from build123d import *

# Parameters (mm, degrees)
BOSS_EXTRUDE1_DEPTH = 5
BOSS_EXTRUDE2_DEPTH = 40
CUT_EXTRUDE1_DEPTH  = 2
CUT_EXTRUDE2_DEPTH  = 370.382836634
FILLET1_R           = 18
FILLET2_R           = 7.5


with BuildPart() as part:
    # Sketch1 → Boss-Extrude1 (new body)
    with BuildSketch(Plane.XY):
        Polygon((67.7, -325.2), (75.2, -325.2), (75.2, -359.2), (-75.2, -359.2), (-75.2, -325.2), (-67.7, -325.2), (-67.7, -345.2), (67.7, -345.2), align=None)
    extrude(amount=-BOSS_EXTRUDE1_DEPTH)

    # Sketch2 → Boss-Extrude2 (add)
    with BuildSketch(Plane(origin=(0, 0, -5), x_dir=(-1, 0, 0), z_dir=(0, 0, -1))):
        Polygon((67.7, -325.2), (75.2, -325.2), (75.2, -359.2), (64.2, -359.2), (64.2, -345.2), (67.7, -345.2), align=None)
        Polygon((-75.2, -359.2), (-75.2, -325.2), (-67.7, -325.2), (-67.7, -345.2), (-64.2, -345.2), (-64.2, -359.2), align=None)
    extrude(amount=BOSS_EXTRUDE2_DEPTH)

    # Sketch3 → Cut-Extrude1 (cut)
    with BuildSketch(Plane(origin=(0, 0, -5), x_dir=(-1, 0, 0), z_dir=(0, 0, -1))):
        with BuildLine():
            Line((-29.2, -347.2), (30.8, -347.2))
            ThreePointArc((30.8, -347.2), (35.8, -352.2), (30.8, -357.2))
            Line((30.8, -357.2), (-29.2, -357.2))
            ThreePointArc((-29.2, -357.2), (-34.2, -352.2), (-29.2, -347.2))
        make_face()
    extrude(amount=-CUT_EXTRUDE1_DEPTH, mode=Mode.SUBTRACT)

    # Sketch4 → Cut-Extrude2 (cut, through all)
    with BuildSketch(Plane(origin=(0, 0, -3), x_dir=(-1, 0, 0), z_dir=(0, 0, -1))):
        with BuildLine():
            Line((-29.2, -349.2), (30.8, -349.2))
            ThreePointArc((30.8, -349.2), (33.8, -352.2), (30.8, -355.2))
            Line((30.8, -355.2), (-29.2, -355.2))
            ThreePointArc((-29.2, -355.2), (-32.2, -352.2), (-29.2, -349.2))
        make_face()
    extrude(amount=-CUT_EXTRUDE2_DEPTH, mode=Mode.SUBTRACT)

    # Fillet1
    fillet1_edges = [part.edges().sort_by_distance(p)[0] for p in [
        (-64.2, -352.2, -5),
        (64.2, -352.2, -5),
    ]]
    fillet(fillet1_edges, radius=FILLET1_R)

    # Fillet2
    fillet2_edges = [part.edges().sort_by_distance(p)[0] for p in [
        (75.2, -325.2, -22.5),
        (-75.2, -325.2, -22.5),
        (-75.2, -359.2, -22.5),
        (75.2, -359.2, -22.5),
    ]]
    fillet(fillet2_edges, radius=FILLET2_R - 0.0001)  # a hair under: the kernel refuses the full size


solid = part.part
Design review of the part built by this model. Coordinates are the model's own, in mm. A direction names the side the tool comes from. Coordinates: 2 decimals unless noted, no trailing zeros. Order: outer loops, then holes, each group sorted by start corner. A loop starts at its lowest first (then second) coordinate and runs counter-clockwise, first axis right, second up. Notation, with made-up numbers: (36.25, 64.25) - (47.25, 64.25) arc R21 cw to (47.25, 85.25) - close; hole circle Ø1 at (17, 40.5). An arc over 180 degrees is marked (long way). Put each result on its own line as item: value.
1) Tool access review of faces 4 (the face through (64.2, -352, -34)), 5 (the face through (34.2, -352.3, -4)), 6 (the face through (-1, -355.2, -2)): name each direction out of +Z, -Z, +X, -X, +Y, -Y from which nothing blocks a thin tool from reaching the whole face with its end or side.
Response values:
face 4: -Z, +Y, -Y
face 5: -Z
face 6: +Z, -Z
2) Take a section at A-A, the plane x = -17. Give the boundary of the cut face in (y, z), and give its area (3 significant figures).
Response values:
outline: (-359.2, -5) - (-357.2, -5) - (-357.2, -3) - (-355.2, -3) - (-355.2, 0) - (-359.2, 0) - close; (-349.2, -3) - (-347.2, -3) - (-347.2, -5) - (-345.2, -5) - (-345.2, 0) - (-349.2, 0) - close
area: 32.0 mm²
3) Take a section at D-D, the plane x = -57. Give the boundary of the cut face in (y, z), and give its area (3 significant figures).
Response values:
outline: (-359.2, -8.6) - (-345.2, -8.6) - (-345.2, 0) - (-359.2, 0) - close
area: 120 mm²
4) Take a section at C-C, the plane y = -329. Give the boundary of the cut face in (x, z), and give its area (3 significant figures).
Response values:
outline: (-74.22, -45) - (-67.7, -45) - (-67.7, 0) - (-74.22, 0) - close; (67.7, -45) - (74.22, -45) - (74.22, 0) - (67.7, 0) - close
area: 587 mm²
5) The part is to be moulded in two halves that separate along X. For faces 1 (the face through (0, -359.2, -2)), 2 (the face through (-35.8, -352.1, -4)), 3 (the face through (-72.945, -357.061, -22.185)), say which applies: released by +X, released by -X, zero draft, split by the parting line, or undercut.
Response values:
face 1: zero draft
face 2: undercut
face 3: released by -X
6) Wall thickness on L1, parallel to X at y = -342, z = -36.5; L2, parallel to X at y = -345.5, z = -27; L3, parallel to Z at x = 0, y = -358: over which ranges is each line inside the solid? List them lowest first. Write a range as from..to.
Response values:
L1: x = -75.2..-67.7, 67.7..75.2
L2: x = -75.2..-64.2, 64.2..75.2
L3: z = -5..0
7) Insertion check: P1, Ø4, axis at x = 23, y = -352, coming from the -Z side; P2, Ø11, axis at y = -354, z = -35.5, coming from the +X side; P3, Ø5, axis at x = 4.5, y = -353, coming from the -Z side; P4, Ø0.6, axis at x = 7.5, z = -4, coming from the +Y side. Each pin has a flat end and moves straight along its axis. Give the tip position at first contact, or say it passes through.
Response values:
P1: passes through
P2: stops at x = 75.2
P3: stops at z = -3
P4: stops at y = -345.2
